CAD build for the part. Positions are in the model's coordinates, mm. A direction names the side the tool comes from. Coordinates: 2 decimals unless noted, no trailing zeros. Loops run counter-clockwise (first coordinate to the right, second up) from the corner with the lowest first, then second, coordinate; pieces in that order, holes last. Notation, with made-up numbers: (-25, -13.5) -> (13, -13.5) arc R20 ccw to (13, -6.5) -> close; hole circle Ø10 at (-33.75, 17). An arc over 180 degrees is marked (long way). Return JSON: item names as keys, results as strings. Group by question number.
(1) Probe L1, parallel to Z at x = 7.62, y = 0.85; L2, parallel to Y at x = 7.62, z = 0.4; L3, parallel to Z at x = 9.75, y = 22.5. List the from-to ranges inside material, lowest first.
(2) Saw through at D-D on z = 15.5. Write the cut outline in (x, y).
(3) Tool access for faces 1 (the face through (8, 1, 21.59)), 2 (the face through (8, 1.27, 13)): list every direction of +Z, -Z, +X, -X, +Y, -Y with a clear straight run to the whole face (end or side of a thin tool).
(4) Saw through at A-A on x = 7.62. Give the number of separate pieces and of enclosed holes in the cut face, then the cut area to 3 significant figures.
(5) Mould opens along X. For faces 3 (the face through (7.33, 0.64, 18.7)), 4 (the face through (8, 0, 11)), 5 (the face through (15.24, 9, 1)) say: pulls with the +X half, pulls with the -X half, needs draft (parallel to the pull), parting line crosses it, or undercut.
(6) Saw through at C-C on x = 1.25. Write the cut outline in (y, z) (3 decimals), then the cut area to 3 significant figures.
(7) Flat gauge pins, fed straight in: pin 1 Ø4 at (x, y) = (12, 9) entering from +Z; pin 2 Ø2 at (x, z) = (5, 17.5) entering from +Y. Where does each tip first touch, or does it go through?
(8) Saw through at B-B on z = 7. Write the cut outline in (x, y).
Autodesk Inventor part; units mm, degrees
ref_plane "YZ Plane" through (0, 0, 0) normal (1, 0, 0) x (0, 1, 0)
ref_plane "XZ Plane" through (0, 0, 0) normal (0, 1, 0) x (-1, 0, 0)
ref_plane "XY Plane" through (0, 0, 0) normal (0, 0, 1) x (1, 0, 0)
sketch "Sketch1" plane through (0, 0, 0) normal (0, 0, 1) x (1, 0, 0)
  line L0 (0, 0) -> (15.24, 0)
  line L1 (15.24, 0) -> (15.24, 25.4)
  line L2 (15.24, 25.4) -> (0, 25.4)
  line L3 (0, 25.4) -> (0, 0)
  dimension "d0" = 25.4
  dimension "d1" = 15.24
extrude "Extrusion1" add sketch "Sketch1" along normal blind 1.27
sketch "Sketch2" plane through (0, 0, 1.27) normal (0, 0, 1) x (1, 0, 0)
  line L0 (15.24, 0) -> (15.24, 25.4)
  line L1 (0, 0) -> (15.24, 0)
  line L2 (15.24, 0) -> (15.24, 1.27)
  line L3 (15.24, 1.27) -> (0, 1.27)
  line L4 (0, 1.27) -> (0, 0)
  dimension "d4" = 1.27
extrude "Extrusion2" add sketch "Sketch2" along normal blind 20.32
sketch "Sketch3" plane through (0, 0, 1.27) normal (0, 0, 1) x (1, 0, 0)
  circle A0 centre (7.62, 19.5834) radius 1.3589
  circle A1 centre (7.62, 9.5758) radius 1.3589
  line L0 (15.24, 1.27) -> (15.24, 25.4)
  line L1 (0, 0) -> (15.24, 0)
  dimension "d7" = 2.7178
  dimension "d8" = 2.7178
  dimension "d9" = 7.62
  dimension "d10" = 7.62
  dimension "d11" = 10.0076
  dimension "d12" = 9.5758
extrude "Extrusion3" cut sketch "Sketch3" against normal blind 25.4
sketch "Sketch4" plane through (0, 1.27, 26.67) normal (0, 1, 0) x (1, 0, 0)
  circle A0 centre (7.62, 19.3065) radius 1.3589
  circle A1 centre (7.62, 9.2989) radius 1.3589
  line L0 (20.32, 1.27) -> (20.32, 25.4)
  line L1 (0, 0) -> (20.32, 0)
  line L2 (15.24, 25.4) -> (15.24, 5.08)
  dimension "d19" = 2.7178
  dimension "d15" = 2.7178
  dimension "d17" = 10.0076
  dimension "d25" = 7.62
  dimension "d26" = 7.62
extrude "Extrusion4" cut sketch "Sketch4" against normal blind 25.4
fillet "Fillet1" radius 3.175 1 edges at (7.62, 1.27, 1.27)
properties part number "Triangle connector"
Geometry results:
{
 "1": {"L1": "0 to 6, 8.72 to 16.01, 18.73 to 21.59", "L2": "0 to 8.22, 10.93 to 18.22, 20.94 to 25.4", "L3": "0 to 1.27"},
 "2": {"outline": "(0, 0) -> (15.24, 0) -> (15.24, 1.27) -> (0, 1.27) -> close"},
 "3": {"face 1": "+Z, +X, -X, +Y, -Y", "face 2": "+Z, +X, -X, +Y"},
 "4": {"separate pieces": "5", "enclosed holes": "0", "area": "46.4 mm²"},
 "5": {"face 3": "undercut", "face 4": "needs draft", "face 5": "pulls with the +X half"},
 "6": {"outline": "(0, 0) -> (25.4, 0) -> (25.4, 1.27) -> (4.445, 1.27) arc R3.175 cw to (1.27, 4.445) -> (1.27, 21.59) -> (0, 21.59) -> close", "area": "60.2 mm²"},
 "7": {"pin 1": "z = 1.27", "pin 2": "y = 1.27"},
 "8": {"outline": "(0, 0) -> (6.31, 0) -> (6.31, 1.27) -> (0, 1.27) -> close; (8.93, 0) -> (15.24, 0) -> (15.24, 1.27) -> (8.93, 1.27) -> close"}
}
